from build123d import *

# Parameters (mm, degrees)
SKETCH1_W           = 53.086
SKETCH1_H           = 42.672
BOSS_EXTRUDE1_DEPTH = 5.334
SKETCH2_W           = 5.334
SKETCH2_H           = 5.588
CUT_EXTRUDE1_DEPTH  = 6.334
SKETCH3_W           = 5.334
SKETCH3_H           = 5.588
CUT_EXTRUDE2_DEPTH  = 6.334
SKETCH4_W           = 5.334
SKETCH4_H           = 5.588
CUT_EXTRUDE3_DEPTH  = 6.334
SKETCH5_W           = 5.334
SKETCH5_H           = 5.588
CUT_EXTRUDE4_DEPTH  = 6.334
SKETCH6_W           = 5.334
SKETCH6_H           = 5.588
CUT_EXTRUDE5_DEPTH  = 6.334
CUT_EXTRUDE6_DEPTH  = 6.334


with BuildPart() as part:
    # Sketch1 → Boss-Extrude1 (new body)
    with BuildSketch(Plane.XY):
        with Locations((26.543, 21.336)):
            Rectangle(SKETCH1_W, SKETCH1_H)
    extrude(amount=BOSS_EXTRUDE1_DEPTH)

    # Sketch2 → Cut-Extrude1 (cut, through all)
    with BuildSketch(Plane.XY.offset(5.334)):
        with Locations((2.667, 39.878)):
            Rectangle(SKETCH2_W, SKETCH2_H)
    extrude(amount=-CUT_EXTRUDE1_DEPTH, mode=Mode.SUBTRACT)

    # Sketch3 → Cut-Extrude2 (cut, through all)
    with BuildSketch(Plane.XY.offset(5.334)):
        with Locations((2.667, 21.336)):
            Rectangle(SKETCH3_W, SKETCH3_H)
    extrude(amount=-CUT_EXTRUDE2_DEPTH, mode=Mode.SUBTRACT)

    # Sketch4 → Cut-Extrude3 (cut, through all)
    with BuildSketch(Plane.XY.offset(5.334)):
        with Locations((2.667, 2.794)):
            Rectangle(SKETCH4_W, SKETCH4_H)
    extrude(amount=-CUT_EXTRUDE3_DEPTH, mode=Mode.SUBTRACT)

    # Sketch5 → Cut-Extrude4 (cut, through all)
    with BuildSketch(Plane.XY.offset(5.334)):
        with Locations((50.419, 39.878)):
            Rectangle(SKETCH5_W, SKETCH5_H)
    extrude(amount=-CUT_EXTRUDE4_DEPTH, mode=Mode.SUBTRACT)

    # Sketch6 → Cut-Extrude5 (cut, through all)
    with BuildSketch(Plane.XY.offset(5.334)):
        with Locations((50.419, 21.336)):
            Rectangle(SKETCH6_W, SKETCH6_H)
        with Locations((50.419, 2.794)):
            Rectangle(SKETCH6_W, SKETCH6_H)
    extrude(amount=-CUT_EXTRUDE5_DEPTH, mode=Mode.SUBTRACT)

    # Sketch11 → Cut-Extrude6 (cut, through all)
    with BuildSketch(Plane.XY.offset(5.334)):
        with BuildLine():
            Line((16.129, 21.336), (16.129, 42.672))
            Line((16.129, 42.672), (36.957, 42.672))
            Line((36.957, 42.672), (36.957, 21.336))
            ThreePointArc((36.957, 21.336), (26.543, 10.922), (16.129, 21.336))
        make_face()
    extrude(amount=-CUT_EXTRUDE6_DEPTH, mode=Mode.SUBTRACT)


solid = part.part
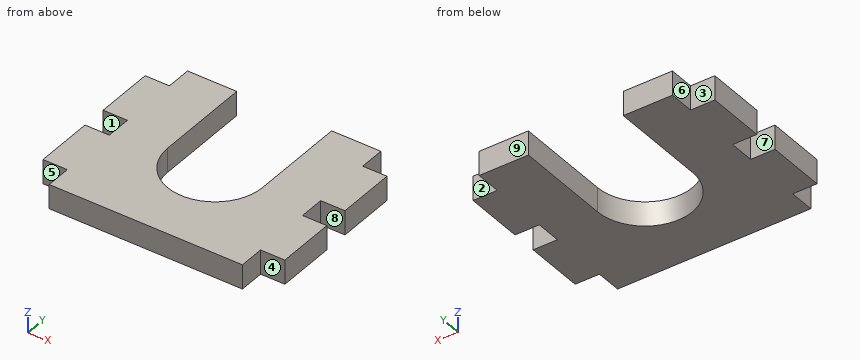
For this review, take the finished solid that the model builds, in its own axes (mm). Face numbers are marked on the shaded views. A direction names the side the tool comes from. Give positions to 0.01 mm unless a question says otherwise; leave off trailing zeros. Loops run counter-clockwise (first coordinate to the right, second up) from the corner with the lowest first, then second, coordinate; pieces in that order, holes last. Notation, with made-up numbers: M 60,-27.75 L 93,-27.75 A14 ccw 93,-19.75 Z; hole C 54.5,-4 d1. An arc over 180 degrees is marked long. Put each result on its own line as item: value. Start each with the question number.
(1) For pin 1 (1.6 mm diameter, centred on y = 2.5, z = 1.5, fed in from +X); pin 2 (1.6 mm diameter, centred on y = 3, z = 1.5, fed in from -X); pin 3 (2.5 mm diameter, centred on x = 49.5, z = 2, fed in from -Y); pin 4 (12 mm diameter, centred on x = 27, y = 25.5, fed in from +Z), all flat-tipped, find the tip position at first contact; note any pin that passes through.
(2) Machinability: for the marked faces 1, 2, 3, 4 and 5, which of the approach directions +Z, -Z, +X, -X, +Y, -Y give a long, thin tool a straight path to every point of the face, cutting with its end or side? Answer none if there is none.
(3) Add section D-D, the plane x = 31.5. Write out the cut boundary in (y, z).
(4) The part is to be moulded in two halves that separate along Y. For the marked faces 6, 7, 8 and 9, say which applies: +Y half, -Y half, draft (parallel to the pull), parting line (faces both ways), or undercut.
(5) Add section A-A, the plane y = 25. Write out the cut boundary in (x, z), then the cut area to 3 significant figures.
(6) Add section C-C, the plane y = 17. Write out the cut boundary in (x, z), then the cut area to 3 significant figures.
(7) Wall thickness on L1, parallel to X at y = 34, z = 0.9; L2, parallel to X at y = 22.5, z = 4.1; L3, parallel to Y at x = 4, z = 2.6: over which ranges is each line inside the solid? List them lowest first.
(8) Add section B-B, the plane z = 4.35. Write out the cut boundary in (x, y), then the cut area to 3 significant figures.
Result:
1. pin 1: stops at x = 47.75
1. pin 2: stops at x = 5.33
1. pin 3: stops at y = 5.59
1. pin 4: passes through
2. face 1: +Z, -Z, -X
2. face 2: +Z, -Z, +X, +Y
2. face 3: +Z, -Z, -X, +Y
2. face 4: +Z, -Z, +X, -Y
2. face 5: +Z, -Z, -X, -Y
3. outline: M 0,0 L 12.18,0 L 12.18,5.33 L 0,5.33 Z
4. face 6: draft
4. face 7: undercut
4. face 8: undercut
4. face 9: +Y half
5. outline: M 0,0 L 16.13,0 L 16.13,5.33 L 0,5.33 Z; M 36.96,0 L 53.09,0 L 53.09,5.33 L 36.96,5.33 Z
5. area: 172 mm^2
6. outline: M 0,0 L 17.07,0 L 17.07,5.33 L 0,5.33 Z; M 36.01,0 L 53.09,0 L 53.09,5.33 L 36.01,5.33 Z
6. area: 182 mm^2
7. L1: x = 0 to 16.13, 36.96 to 53.09
7. L2: x = 5.33 to 16.13, 36.96 to 47.75
7. L3: y = 5.59 to 18.54, 24.13 to 37.08
8. outline: M 0,5.59 L 5.33,5.59 L 5.33,0 L 47.75,0 L 47.75,5.59 L 53.09,5.59 L 53.09,18.54 L 47.75,18.54 L 47.75,24.13 L 53.09,24.13 L 53.09,37.08 L 47.75,37.08 L 47.75,42.67 L 36.96,42.67 L 36.96,21.34 A10.41 cw 16.13,21.34 L 16.13,42.67 L 5.33,42.67 L 5.33,37.08 L 0,37.08 L 0,24.13 L 5.33,24.13 L 5.33,18.54 L 0,18.54 Z
8. area: 1,470 mm^2
